Answer from the drawing. Dimensions are ordinates in mm from the lowest x, y and z of the part. A direction names the side the tool comes from. Round coordinates to 2 decimals unless told otherwise and drop trailing zeros. Order: outer loops, then holes, each group sorted by start corner. A loop starts at its lowest first (then second) coordinate and runs counter-clockwise, first axis right, second up. Notation, with made-up numbers: M 20,54.5 L 50,54.5 A20 cw 50,71.5 Z; hole C 7,17 d11. An arc over 180 degrees is marked long. Use one line per item in the form item = value. Start each with the question number.
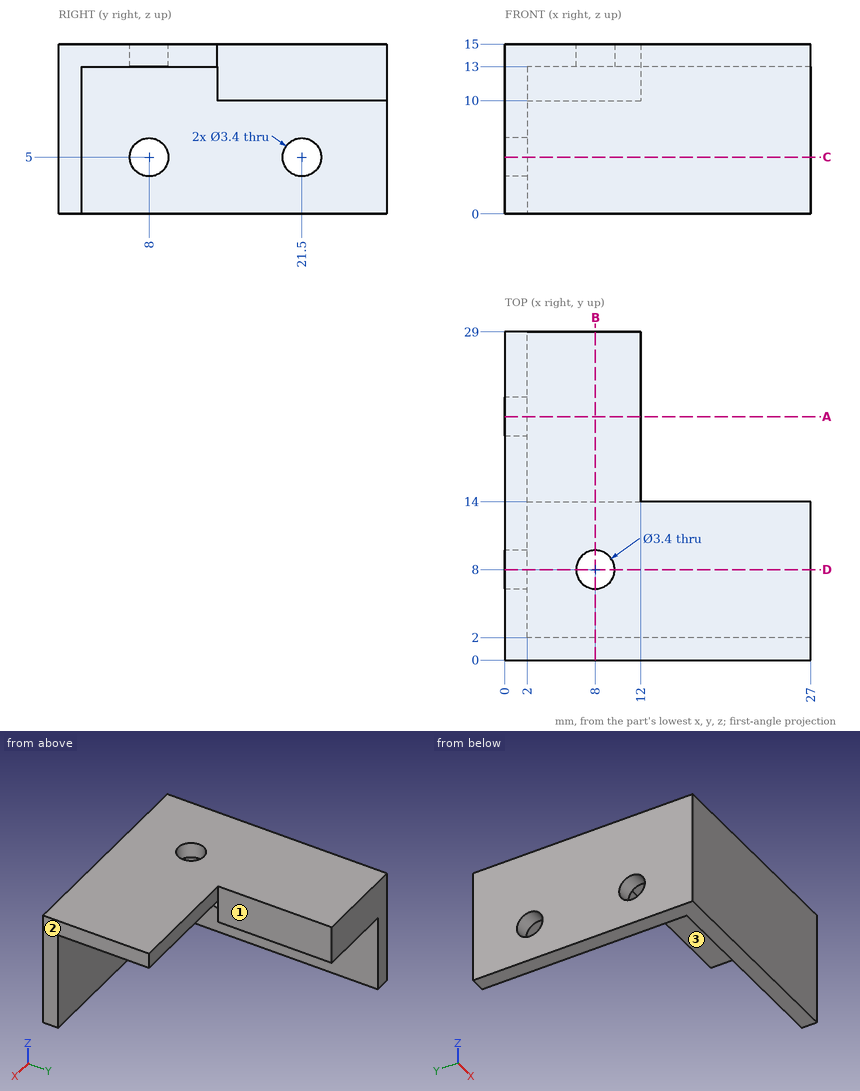
Item 1: Section D-D (y = 8) is taken. Write down the section's boundary in (x, z), and give its area (3 significant figures).
Item 2: Section B-B (x = 8) is taken. Write down the section's boundary in (y, z).
Item 3: Section C-C (z = 5) is taken. Write down the section's boundary in (x, y).
Item 4: Find the intervals of material crossed by L1, parallel to Z at x = 1.4, y = 21.5; L2, parallel to Y at x = 6.25, z = 12; L3, parallel to X at y = 12, z = 9.25, in increasing order. Write a range as [from, to].
Item 5: A tool of negligible diameter and unlimited length cuts with its end or side. For the marked faces 1, 2 and 3, from which of +Z, -Z, +X, -X, +Y, -Y can it reach the whole face along a straight path? Write none if from no direction.
Item 6: Section A-A (y = 21.5) is taken. Write down the section's boundary in (x, z).
Item 7: Given P1, Ø6, axis at x = 16, z = 2.5, coming from the +Y side; P2, Ø8, axis at x = 15, y = 11, coming from the -Z side; P3, Ø5.5, axis at y = 21.5, z = 5, coming from the +X side, each flat-ended and moving along its own axis, determine where each tip first touches the part or whether it passes through.
The answers:
q1.outline = M 0,0 L 2,0 L 2,3.3 L 0,3.3 Z; M 0,6.7 L 2,6.7 L 2,13 L 6.3,13 L 6.3,15 L 0,15 Z; M 9.7,13 L 27,13 L 27,15 L 9.7,15 Z
q1.area = 66.4 mm²
q2.outline = M 0,0 L 2,0 L 2,13 L 6.3,13 L 6.3,15 L 0,15 Z; M 9.7,13 L 14,13 L 14,10 L 29,10 L 29,15 L 9.7,15 Z
q3.outline = M 0,0 L 27,0 L 27,2 L 2,2 L 2,6.3 L 0,6.3 Z; M 0,9.7 L 2,9.7 L 2,19.8 L 0,19.8 Z; M 0,23.2 L 2,23.2 L 2,29 L 0,29 Z
q4.L1 = [0, 3.3], [6.7, 15]
q4.L2 = [0, 2], [14, 29]
q4.L3 = [0, 2]
q5.face_1 = +Z, -Z, +X, +Y
q5.face_2 = +Z, -Z, +X, +Y, -Y
q5.face_3 = -Z, +X
q6.outline = M 0,0 L 2,0 L 2,3.3 L 0,3.3 Z; M 0,6.7 L 2,6.7 L 2,10 L 12,10 L 12,15 L 0,15 Z
q7.P1 = 2
q7.P2 = 13
q7.P3 = 2
